Design review of the part built by this model. Coordinates are the model's own, in mm. A direction names the side the tool comes from. Coordinates: 2 decimals unless noted, no trailing zeros. Loops run counter-clockwise (first coordinate to the right, second up) from the corner with the lowest first, then second, coordinate; pieces in that order, holes last. Notation, with made-up numbers: (-25.75, 9) -> (8.25, 9) arc R17 cw to (8.25, 28) -> close; hole circle Ø4 at (3, 53.25). An arc over 180 degrees is marked (long way). Use CSV: the item, a comma, the result in double quotes.
```python
from build123d import *

# Parameters (mm, degrees)
SKETCH2_W           = 6.35
SKETCH2_H           = 44.45
SKETCH2_W_2         = 20.864285714
SKETCH2_H_2         = 6.35
SKETCH2_W_3         = 27.214285714
BOSS_EXTRUDE1_DEPTH = 6.35
SKETCH3_W           = 7.9375
SKETCH3_H           = 228.6
CUT_EXTRUDE1_DEPTH  = 186.241592252
SKETCH4_R           = 3.175
CUT_EXTRUDE2_DEPTH  = 186.241592252
SKETCH5_R           = 1.5
CUT_EXTRUDE3_DEPTH  = 6.35
SKETCH6_W           = 6.35
SKETCH6_H           = 44.45
BOSS_EXTRUDE2_DEPTH = 6.35
SKETCH7_W           = 27.214285714
SKETCH7_H           = 6.35
CUT_EXTRUDE4_DEPTH  = 6.35
SKETCH9_W           = 6.35
SKETCH9_H           = 222.25
SKETCH9_W_2         = 20.864285714
SKETCH9_H_2         = 6.35
CUT_EXTRUDE5_DEPTH  = 6.35


with BuildPart() as part:
    # Sketch2 → Boss-Extrude1 (new body)
    with BuildSketch(Plane.XY):
        Polygon((0, -152.4), (0, 152.4), (-88.9, 152.4), (-88.9, 107.95), (-88.9, 63.5), (-88.9, 19.05), (-88.9, -25.4), (-88.9, -69.85), (-88.9, -114.3), (-88.9, -152.4), (-68.035714286, -152.4), (-40.821428571, -152.4), (-13.607142857, -152.4), align=None)
        Polygon((88.9, 152.4), (0, 152.4), (0, -152.4), (13.607142857, -152.4), (40.821428571, -152.4), (68.035714286, -152.4), (88.9, -152.4), (88.9, -114.3), (88.9, -69.85), (88.9, -25.4), (88.9, 19.05), (88.9, 63.5), (88.9, 107.95), align=None)
        with Locations((-92.075, 85.725)):
            Rectangle(SKETCH2_W, SKETCH2_H)
        with Locations((-92.075, -3.175)):
            Rectangle(SKETCH2_W, SKETCH2_H)
        with Locations((-92.075, -92.075)):
            Rectangle(SKETCH2_W, SKETCH2_H)
        with Locations((-78.467857143, -155.575)):
            Rectangle(SKETCH2_W_2, SKETCH2_H_2)
        with Locations((-27.214285714, -155.575)):
            Rectangle(SKETCH2_W_3, SKETCH2_H_2)
        with Locations((27.214285714, -155.575)):
            Rectangle(SKETCH2_W_3, SKETCH2_H_2)
        with Locations((92.075, -92.075)):
            Rectangle(SKETCH2_W, SKETCH2_H)
        with Locations((92.075, -3.175)):
            Rectangle(SKETCH2_W, SKETCH2_H)
        with Locations((92.075, 85.725)):
            Rectangle(SKETCH2_W, SKETCH2_H)
        with Locations((78.467857143, -155.575)):
            Rectangle(SKETCH2_W_2, SKETCH2_H_2)
    extrude(amount=BOSS_EXTRUDE1_DEPTH)

    # Sketch3 → Cut-Extrude1 (cut, through all)
    with BuildSketch(Plane.XY.offset(6.35)):
        with Locations((0, 38.1)):
            Rectangle(SKETCH3_W, SKETCH3_H)
    extrude(amount=-CUT_EXTRUDE1_DEPTH, mode=Mode.SUBTRACT)

    # Sketch4 → Cut-Extrude2 (cut, through all)
    with BuildSketch(Plane.XY.offset(6.35)):
        with Locations((-50.8, -139.7)):
            Circle(SKETCH4_R)
    extrude(amount=-CUT_EXTRUDE2_DEPTH, mode=Mode.SUBTRACT)

    # Sketch5 → Cut-Extrude3 (cut)
    with BuildSketch(Plane.XY.offset(6.35)):
        with Locations((-76.2, 137.4)):
            Circle(SKETCH5_R)
        with Locations((-76.2, 121.65)):
            Circle(SKETCH5_R)
        with Locations((76.2, 121.65)):
            Circle(SKETCH5_R)
        with Locations((76.2, 137.4)):
            Circle(SKETCH5_R)
    extrude(amount=-CUT_EXTRUDE3_DEPTH, mode=Mode.SUBTRACT)

    # Sketch6 → Boss-Extrude2 (add)
    with BuildSketch(Plane.XY.offset(6.35)):
        with Locations((-92.075, 41.275)):
            Rectangle(SKETCH6_W, SKETCH6_H)
        with Locations((-92.075, -47.625)):
            Rectangle(SKETCH6_W, SKETCH6_H)
        with Locations((92.075, 41.275)):
            Rectangle(SKETCH6_W, SKETCH6_H)
        with Locations((92.075, -47.625)):
            Rectangle(SKETCH6_W, SKETCH6_H)
    extrude(amount=-BOSS_EXTRUDE2_DEPTH)

    # Sketch7 → Cut-Extrude4 (cut)
    with BuildSketch(Plane.XY.offset(6.35)):
        with Locations((-27.214285714, -155.575)):
            Rectangle(SKETCH7_W, SKETCH7_H)
        with Locations((27.214285714, -155.575)):
            Rectangle(SKETCH7_W, SKETCH7_H)
    extrude(amount=-CUT_EXTRUDE4_DEPTH, mode=Mode.SUBTRACT)

    # Sketch9 → Cut-Extrude5 (cut)
    with BuildSketch(Plane(origin=(0, 0, 0), x_dir=(-1, 0, 0), z_dir=(0, 0, -1))):
        with Locations((-92.075, -3.175)):
            Rectangle(SKETCH9_W, SKETCH9_H)
        with Locations((92.075, -3.175)):
            Rectangle(SKETCH9_W, SKETCH9_H)
        with Locations((-78.467857143, -155.575)):
            Rectangle(SKETCH9_W_2, SKETCH9_H_2)
        with Locations((78.467857143, -155.575)):
            Rectangle(SKETCH9_W_2, SKETCH9_H_2)
    extrude(amount=-CUT_EXTRUDE5_DEPTH, mode=Mode.SUBTRACT)


solid = part.part
```
Item 1: To check wall thickness, follow line 1 along Y through (x, z) = (-76.2, 2); line 2 along X through (y, z) = (-139.7, 4.5) (3 decimals); line 3 along X through (y, z) = (121.65, 4.5). State the ranges of each line that lie inside material, in increasing order.
Checked values:
line 1,"-152.4 to 120.15, 123.15 to 135.9, 138.9 to 152.4"
line 2,"-88.9 to -53.975, -47.625 to 88.9"
line 3,"-88.9 to -77.7, -74.7 to -3.97, 3.97 to 74.7, 77.7 to 88.9"
Item 2: Draft analysis for pull direction X (two halves, no side actions). For faces 1 (the face through (-88.9, -2, 3)), 2 (the face through (88.9, -2, 3)), 3 (the face through (0, -76.2, 3)), 4 (the face through (-21, 2, 0)), state which applies: pulls with the +X half, pulls with the -X half, needs draft (parallel to the pull), parting line crosses it, or undercut.
Checked values:
face 1,"pulls with the -X half"
face 2,"pulls with the +X half"
face 3,"undercut"
face 4,"needs draft"
Item 3: Machinability: for faces 5 (the face through (-3.969, 36, 3)), 6 (the face through (1, -152.4, 3)), which of the approach directions +Z, -Z, +X, -X, +Y, -Y give a long, thin tool a straight path to every point of the face, cutting with its end or side? Answer none if there is none.
Checked values:
face 5,"+Z, -Z, +Y"
face 6,"+Z, -Z, +X, -X, -Y"
Item 4: Add section A-A (y = -139.7). Give the boundary of the cut face in (x, z) (3 decimals).
Checked values:
outline,"(-88.9, 0) -> (-53.975, 0) -> (-53.975, 6.35) -> (-88.9, 6.35) -> close; (-47.625, 0) -> (88.9, 0) -> (88.9, 6.35) -> (-47.625, 6.35) -> close"
Item 5: Add section C-C (y = 82). Give the boundary of the cut face in (x, z).
Checked values:
outline,"(-88.9, 0) -> (-3.97, 0) -> (-3.97, 6.35) -> (-88.9, 6.35) -> close; (3.97, 0) -> (88.9, 0) -> (88.9, 6.35) -> (3.97, 6.35) -> close"
Item 6: Add section B-B (z = 4.5). Give the boundary of the cut face in (x, y) (3 decimals), then the cut area to 3 significant figures.
Checked values:
outline,"(-88.9, -152.4) -> (88.9, -152.4) -> (88.9, 152.4) -> (3.969, 152.4) -> (3.969, -76.2) -> (-3.969, -76.2) -> (-3.969, 152.4) -> (-88.9, 152.4) -> close; hole circle Ø3 at (-76.2, 121.65); hole circle Ø3 at (-76.2, 137.4); hole circle Ø6.35 at (-50.8, -139.7); hole circle Ø3 at (76.2, 121.65); hole circle Ø3 at (76.2, 137.4)"
area,"52,300 mm^2"
